Input: part model. Units: mm. Frame: model coordinates. A direction names the side the tool comes from. Round coordinates to 2 decimals unless told otherwise and drop trailing zeros. Loops run counter-clockwise (first coordinate to the right, second up) from the corner with the lowest first, then second, coordinate; pieces in that order, holes last. Notation, with made-up numbers: (-18.5, -7) -> (39.5, -7) arc R34 cw to (39.5, 28) -> close; hole circle Ø4 at (44, 57). An arc over 180 degrees is marked (long way). Answer as a JSON object with one key per item and string values.
```python
from build123d import *

# Parameters (mm, degrees)
SKETCH_1_W               = 1.74
SKETCH_1_H               = 1.74
SKETCH_1_W_2             = 3
SKETCH_1_H_2             = 3
EXTRUDE_1_DEPTH          = 24
CUT_EXTRUDE_1_DEPTH      = 28.241328896
CUT_EXTRUDE_1_DEPTH_BACK = 28.241328896
SKETCH_2_W               = 16
SKETCH_2_H               = 10


with BuildPart() as part:
    # 草图1 → 凸台-拉伸1 (new body)
    # profile 1 of 2: a face of its own
    with BuildSketch(Plane(origin=(0, 0, 0), x_dir=(0, 0, -1), z_dir=(1, 0, 0))):
        Polygon((0.5, 1.5), (0.5, 9.8), (1.5, 9.8), (1.5, 12.8), (-1.5, 12.8), (-1.5, 9.8), (-0.5, 9.8), (-0.5, 1.5), align=None)
        with Locations((0, 11.3)):
            Rectangle(SKETCH_1_W, SKETCH_1_H, mode=Mode.SUBTRACT)
    # profile 2 of 2: a face of its own
    with BuildSketch(Plane(origin=(0, 0, 0), x_dir=(0, 0, -1), z_dir=(1, 0, 0))):
        Rectangle(SKETCH_1_W_2, SKETCH_1_H_2)
        Rectangle(SKETCH_1_W, SKETCH_1_H, mode=Mode.SUBTRACT)
    extrude(amount=EXTRUDE_1_DEPTH)

    # 草图2 → 切除-拉伸1 (cut, two sides: drawn at the far end of the back side and taken through both)
    with BuildSketch(Plane.XY.offset(-CUT_EXTRUDE_1_DEPTH_BACK)):
        with Locations((12, 12.8)):
            Rectangle(SKETCH_2_W, SKETCH_2_H)
        with Locations((12, -1.5)):
            Rectangle(SKETCH_2_W, SKETCH_2_H)
    extrude(amount=CUT_EXTRUDE_1_DEPTH + CUT_EXTRUDE_1_DEPTH_BACK, mode=Mode.SUBTRACT)


solid = part.part
```
1) Section A-A, the plane z = 1.1. Output: boundary loops of the cut face in (x, y).
Output:
{"outline": "(0, -1.5) -> (4, -1.5) -> (4, 1.5) -> (0, 1.5) -> close; (0, 9.8) -> (4, 9.8) -> (4, 12.8) -> (0, 12.8) -> close; (20, -1.5) -> (24, -1.5) -> (24, 1.5) -> (20, 1.5) -> close; (20, 9.8) -> (24, 9.8) -> (24, 12.8) -> (20, 12.8) -> close"}
2) Section C-C, the plane y = 2.75. Output: boundary loops of the cut face in (x, z), plus the area to 3 significant figures.
Output:
{"outline": "(0, -0.5) -> (4, -0.5) -> (4, 0.5) -> (0, 0.5) -> close; (20, -0.5) -> (24, -0.5) -> (24, 0.5) -> (20, 0.5) -> close", "area": "8.00 mm^2"}
3) Section D-D, the plane y = 5.5. Output: boundary loops of the cut face in (x, z), plus the area to 3 significant figures.
Output:
{"outline": "(0, -0.5) -> (24, -0.5) -> (24, 0.5) -> (0, 0.5) -> close", "area": "24.0 mm^2"}
4) Ray query, probe 1 along Y at (x, z) = (21, -0.3); probe 2 along Y at (x, z) = (22.75, -1.05); probe 3 along X at (y, z) = (11.75, 1.25). Return the intervals inside material, ascending.
Output:
{"probe 1": "y = -1.5 to -0.87, 0.87 to 10.43, 12.17 to 12.8", "probe 2": "y = -1.5 to 1.5, 9.8 to 12.8", "probe 3": "x = 0 to 4, 20 to 24"}
5) Draft query along Y for faces 4 (the face through (2, 12.8, 0)), 5 (the face through (2, 11, 0.87)), 6 (the face through (2, 11, -1.5)). Return one class per face: +Y half, -Y half, draft (parallel to the pull), parting line (faces both ways), or undercut.
Output:
{"face 4": "+Y half", "face 5": "undercut", "face 6": "draft"}
6) Reachability of faces 1 (the face through (12, 6, 0.5)), 2 (the face through (22, 1.5, -1)), 3 (the face through (2, 0, 0.87)) from +Z, -Z, +X, -X, +Y, -Y: full face, straight path, thin tool, end or side. Return the list, or none.
Output:
{"face 1": "+Z, +X, -X", "face 2": "-Z, +X, -X", "face 3": "+X, -X"}
7) Contact query for flat-ended pins moving along their axis: P1, Ø0.9, axis at y = 0, z = 0, coming from the +X side; P2, Ø0.8, axis at x = 11, z = 0, coming from the +Y side; P3, Ø6.5, axis at x = 13.5, y = 4, coming from the -Z side. Output: stop coordinate, or through.
Output:
{"P1": "passes through", "P2": "stops at y = 7.8", "P3": "stops at z = -0.5"}
8) Section B-B, the plane x = 1.75. Output: boundary loops of the cut face in (y, z), plus the area to 3 significant figures.
Output:
{"outline": "(-1.5, -1.5) -> (1.5, -1.5) -> (1.5, -0.5) -> (9.8, -0.5) -> (9.8, -1.5) -> (12.8, -1.5) -> (12.8, 1.5) -> (9.8, 1.5) -> (9.8, 0.5) -> (1.5, 0.5) -> (1.5, 1.5) -> (-1.5, 1.5) -> close; hole (-0.87, -0.87) -> (0.87, -0.87) -> (0.87, 0.87) -> (-0.87, 0.87) -> close; hole (10.43, -0.87) -> (12.17, -0.87) -> (12.17, 0.87) -> (10.43, 0.87) -> close", "area": "20.2 mm^2"}
